The model under review builds one solid part; all positions refer to its coordinate system, in mm. Face numbers are marked on the shaded views. A direction names the side the tool comes from. Round coordinates to 2 decimals unless told otherwise and drop trailing zeros. Write each loop counter-clockwise with the first axis right and the second up, starting at its lowest first coordinate (ties: lowest second). Pieces come first, ordered by that corner, then holes. Notation, with made-up numbers: (-18.5, 52) -> (9.5, 52) arc R20 ccw to (9.5, 89) -> close; hole circle Ø6 at (-40, 57.25). An arc over 180 degrees is marked (long way). Answer as a JSON object with one key per item and string values. Group by question number.
1) To check wall thickness, follow probe 1 along X at (y, z) = (-14.5, 26); probe 2 along X at (y, z) = (-7, 34); probe 3 along X at (y, z) = (-9.5, 32). State the ranges of each line that lie inside material, in increasing order. Write a range as [from, to].
2) We need section B-B, the plane x = -68. Write out the cut boundary in (y, z), then the cut area to 3 significant figures.
3) Mouldability with a two-part tool opening along X and no side actions: class the marked faces 1, 2 and 3 as pulls with the +X half, pulls with the -X half, needs draft (parallel to the pull), parting line crosses it, or undercut.
4) We need section A-A, the plane z = -8. Write out the cut boundary in (x, y).
5) Machinability: for the marked faces 4 and 5, which of the approach directions +Z, -Z, +X, -X, +Y, -Y give a long, thin tool a straight path to every point of the face, cutting with its end or side? Answer none if there is none.
6) Insertion check: pin 1 Ø12 at (y, z) = (2.5, 37) entering from -X; pin 2 Ø6 at (y, z) = (-2.5, 6) entering from +X; pin 3 Ø8 at (x, z) = (-57.5, -28) entering from +Y. Each pin has a flat end and moves straight along its axis. Give the tip position at first contact, or say it passes through.
7) We need section C-C, the plane x = 32.5. Write out the cut boundary in (y, z).
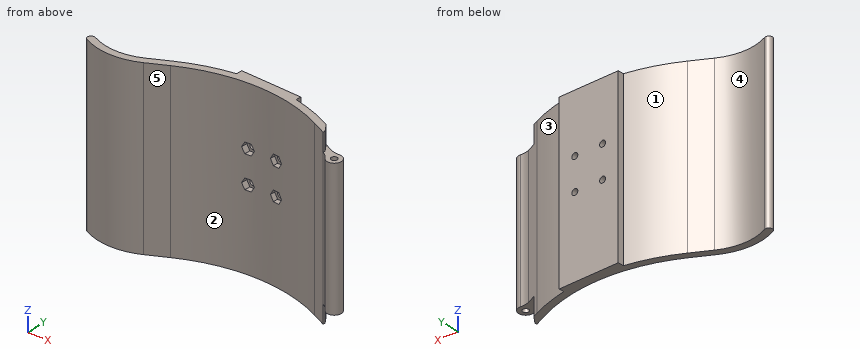
from build123d import *

# Parameters (mm, degrees)
CROQUIS1_R                   = 1.7
SALIENTE_EXTRUIR1_DEPTH      = 48
REDONDEO1_R                  = 10
CORTAR_EXTRUIR1_DEPTH        = 10
CHAFL_N1_SIZE                = 3
CHAFL_N1_SIZE2               = 5.196152423
CHAFL_N1_PART_2_SIZE         = 3
CHAFL_N1_PART_2_SIZE2        = 5.196152423
SALIENTE_EXTRUIR2_DEPTH      = 48
SALIENTE_EXTRUIR2_DEPTH_BACK = 48
CORTAR_EXTRUIR3_REACH        = 30.364
CROQUIS6_R                   = 1.7
CORTAR_EXTRUIR4_REACH        = 27.364


with BuildPart() as part:
    # Croquis1 → Saliente-Extruir1 (new body, symmetric)
    with BuildSketch(Plane.XY):
        with BuildLine():
            Line((-39.737417582, -9.247677161), (-50.50439396, -14.545999505))
            ThreePointArc((-50.50439396, -14.545999505), (-66.386844231, -18.110333527), (-82.148948738, -14.04674335))
            ThreePointArc((-82.148948738, -14.04674335), (-82.975471065, -11.341773693), (-80.270501408, -10.515251366))
            ThreePointArc((-80.270501408, -10.515251366), (-66.323744082, -14.110831262), (-52.270501408, -10.957007379))
            Line((-52.270501408, -10.957007379), (-41.50352503, -5.658685035))
            ThreePointArc((-41.50352503, -5.658685035), (0, 4), (41.50352503, -5.658685035))
            Line((41.50352503, -5.658685035), (52.270501408, -10.957007379))
            ThreePointArc((52.270501408, -10.957007379), (58.084598166, -16.047104806), (50.50439396, -14.545999505))
            Line((50.50439396, -14.545999505), (39.737417582, -9.247677161))
            ThreePointArc((39.737417582, -9.247677161), (0, 0), (-39.737417582, -9.247677161))
        make_face()
        with Locations((54.49560604, -14.280997358)):
            Circle(CROQUIS1_R, mode=Mode.SUBTRACT)
    extrude(amount=SALIENTE_EXTRUIR1_DEPTH, both=True)

    # Redondeo1
    redondeo1_edges = [part.edges().sort_by_distance(p)[0] for p in [
        (52.270501408, -10.957007379, 0),
        (50.50439396, -14.545999505, 0),
    ]]
    fillet(redondeo1_edges, radius=REDONDEO1_R)

    # Croquis3 → Cortar-Extruir1 (cut)
    with BuildSketch(Plane.XY.offset(48)):
        with BuildLine():
            Line((48.908512195, -9.302605814), (47.142404747, -12.89159794))
            ThreePointArc((47.142404747, -12.89159794), (49.37979166, -14.398010057), (51.133186064, -16.4475919))
            ThreePointArc((51.133186064, -16.4475919), (58.084598166, -16.047104806), (54.160798833, -10.295033969))
            ThreePointArc((54.160798833, -10.295033969), (51.467117745, -10.156254046), (48.908512195, -9.302605814))
        make_face()
    cortar_extruir1 = extrude(amount=-CORTAR_EXTRUIR1_DEPTH, mode=Mode.SUBTRACT)

    # Simetría1: Cortar-Extruir1 across plane
    add(cortar_extruir1.mirror(Plane.XY), mode=Mode.SUBTRACT)

    # Chaflán1
    chafl_n1_edges = [part.edges().sort_by_distance(p)[0] for p in [
        (48.908512195, -9.302605814, 43),
    ]]
    chafl_n1_side = [part.faces().sort_by_distance(p)[0] for p in [
        (48.025458471, -11.097101877, 43),
    ]]
    chamfer(chafl_n1_edges, length=CHAFL_N1_SIZE, length2=CHAFL_N1_SIZE2, reference=chafl_n1_side[0])

    # Chaflán1 part 2
    chafl_n1_part_2_edges = [part.edges().sort_by_distance(p)[0] for p in [
        (48.908512195, -9.302605814, -43),
    ]]
    chafl_n1_part_2_side = [part.faces().sort_by_distance(p)[0] for p in [
        (48.025458471, -11.097101877, -43),
    ]]
    chamfer(chafl_n1_part_2_edges, length=CHAFL_N1_PART_2_SIZE, length2=CHAFL_N1_PART_2_SIZE2, reference=chafl_n1_part_2_side[0])

    # Croquis5 → Saliente-Extruir2 (add, two sides)
    with BuildSketch(Plane.XY) as saliente_extruir2_sk:
        with BuildLine():
            Line((-12.976702091, 6.440682618), (20.976702091, 4.661260106))
            Line((20.976702091, 4.661260106), (20.819694222, 1.665371501))
            ThreePointArc((20.819694222, 1.665371501), (3.897584771, 3.91916116), (-13.153078528, 3.075219716))
            Line((-13.153078528, 3.075219716), (-12.976702091, 6.440682618))
        make_face()
    extrude(amount=SALIENTE_EXTRUIR2_DEPTH)
    extrude(saliente_extruir2_sk.sketch, amount=-SALIENTE_EXTRUIR2_DEPTH_BACK)

    # Croquis6 → Cortar-Extruir3 (cut, up to next)
    with BuildSketch(Plane(origin=(0.301073462, 5.744823887, 0), x_dir=(0.998629535, -0.052335956, 0), z_dir=(0.052335956, 0.998629535, 0)), mode=Mode.PRIVATE) as cortar_extruir3_sk1:
        with Locations((-4.295997255, 3)):
            Circle(CROQUIS6_R)
    cortar_extruir3_tool1 = extrude(cortar_extruir3_sk1.sketch, amount=-CORTAR_EXTRUIR3_REACH, mode=Mode.PRIVATE) & part.part
    add(cortar_extruir3_tool1.solids().sort_by_distance((-3.989036, 5.969659, -3))[0], mode=Mode.SUBTRACT)
    # Croquis6 → Cortar-Extruir3 (cut, up to next)
    with BuildSketch(Plane(origin=(0.301073462, 5.744823887, 0), x_dir=(0.998629535, -0.052335956, 0), z_dir=(0.052335956, 0.998629535, 0)), mode=Mode.PRIVATE) as cortar_extruir3_sk2:
        with Locations((11.704002745, 3)):
            Circle(CROQUIS6_R)
    cortar_extruir3_tool2 = extrude(cortar_extruir3_sk2.sketch, amount=-CORTAR_EXTRUIR3_REACH, mode=Mode.PRIVATE) & part.part
    add(cortar_extruir3_tool2.solids().sort_by_distance((11.989036, 5.132284, -3))[0], mode=Mode.SUBTRACT)
    # Croquis6 → Cortar-Extruir3 (cut, up to next)
    with BuildSketch(Plane(origin=(0.301073462, 5.744823887, 0), x_dir=(0.998629535, -0.052335956, 0), z_dir=(0.052335956, 0.998629535, 0)), mode=Mode.PRIVATE) as cortar_extruir3_sk3:
        with Locations((11.704002745, -15)):
            Circle(CROQUIS6_R)
    cortar_extruir3_tool3 = extrude(cortar_extruir3_sk3.sketch, amount=-CORTAR_EXTRUIR3_REACH, mode=Mode.PRIVATE) & part.part
    add(cortar_extruir3_tool3.solids().sort_by_distance((11.989036, 5.132284, 15))[0], mode=Mode.SUBTRACT)
    # Croquis6 → Cortar-Extruir3 (cut, up to next)
    with BuildSketch(Plane(origin=(0.301073462, 5.744823887, 0), x_dir=(0.998629535, -0.052335956, 0), z_dir=(0.052335956, 0.998629535, 0)), mode=Mode.PRIVATE) as cortar_extruir3_sk4:
        with Locations((-4.295997255, -15)):
            Circle(CROQUIS6_R)
    cortar_extruir3_tool4 = extrude(cortar_extruir3_sk4.sketch, amount=-CORTAR_EXTRUIR3_REACH, mode=Mode.PRIVATE) & part.part
    add(cortar_extruir3_tool4.solids().sort_by_distance((-3.989036, 5.969659, 15))[0], mode=Mode.SUBTRACT)

    # Croquis7 → Cortar-Extruir4 (cut, up to next)
    with BuildSketch(Plane(origin=(0.144065594, 2.748935283, 0), x_dir=(0.998629535, -0.052335956, 0), z_dir=(0.052335956, 0.998629535, 0)), mode=Mode.PRIVATE) as cortar_extruir4_sk1:
        Polygon((-0.889630667, 3), (-2.592813961, 5.95), (-5.999180549, 5.95), (-7.702363843, 3), (-5.999180549, 0.05), (-2.592813961, 0.05), align=None)
    cortar_extruir4_tool1 = extrude(cortar_extruir4_sk1.sketch, amount=-CORTAR_EXTRUIR4_REACH, mode=Mode.PRIVATE) & part.part
    add(cortar_extruir4_tool1.solids().sort_by_distance((-4.146044, 2.97377, -3))[0], mode=Mode.SUBTRACT)
    # Croquis7 → Cortar-Extruir4 (cut, up to next)
    with BuildSketch(Plane(origin=(0.144065594, 2.748935283, 0), x_dir=(0.998629535, -0.052335956, 0), z_dir=(0.052335956, 0.998629535, 0)), mode=Mode.PRIVATE) as cortar_extruir4_sk2:
        Polygon((15.110369333, 3), (13.407186039, 5.95), (10.000819451, 5.95), (8.297636157, 3), (10.000819451, 0.05), (13.407186039, 0.05), align=None)
    cortar_extruir4_tool2 = extrude(cortar_extruir4_sk2.sketch, amount=-CORTAR_EXTRUIR4_REACH, mode=Mode.PRIVATE) & part.part
    add(cortar_extruir4_tool2.solids().sort_by_distance((11.832028, 2.136395, -3))[0], mode=Mode.SUBTRACT)
    # Croquis7 → Cortar-Extruir4 (cut, up to next)
    with BuildSketch(Plane(origin=(0.144065594, 2.748935283, 0), x_dir=(0.998629535, -0.052335956, 0), z_dir=(0.052335956, 0.998629535, 0)), mode=Mode.PRIVATE) as cortar_extruir4_sk3:
        Polygon((-0.889630667, -15), (-2.592813961, -12.05), (-5.999180549, -12.05), (-7.702363843, -15), (-5.999180549, -17.95), (-2.592813961, -17.95), align=None)
    cortar_extruir4_tool3 = extrude(cortar_extruir4_sk3.sketch, amount=-CORTAR_EXTRUIR4_REACH, mode=Mode.PRIVATE) & part.part
    add(cortar_extruir4_tool3.solids().sort_by_distance((-4.146044, 2.97377, 15))[0], mode=Mode.SUBTRACT)
    # Croquis7 → Cortar-Extruir4 (cut, up to next)
    with BuildSketch(Plane(origin=(0.144065594, 2.748935283, 0), x_dir=(0.998629535, -0.052335956, 0), z_dir=(0.052335956, 0.998629535, 0)), mode=Mode.PRIVATE) as cortar_extruir4_sk4:
        Polygon((15.110369333, -15), (13.407186039, -12.05), (10.000819451, -12.05), (8.297636157, -15), (10.000819451, -17.95), (13.407186039, -17.95), align=None)
    cortar_extruir4_tool4 = extrude(cortar_extruir4_sk4.sketch, amount=-CORTAR_EXTRUIR4_REACH, mode=Mode.PRIVATE) & part.part
    add(cortar_extruir4_tool4.solids().sort_by_distance((11.832028, 2.136395, 15))[0], mode=Mode.SUBTRACT)


solid = part.part
Here are the results:
{
 "1": {"probe 1": "x = [-81.27, -50.41], [49.49, 52.81], [56.18, 58.49]", "probe 2": "x = [-44.23, -34.8], [34.8, 44.23]", "probe 3": "x = [-49.31, -40.25], [40.25, 49.33]"},
 "2": {"outline": "(-18.05, -48) -> (-14.04, -48) -> (-14.04, 48) -> (-18.05, 48) -> close", "area": "385 mm^2"},
 "3": {"face 1": "pulls with the -X half", "face 2": "undercut", "face 3": "pulls with the +X half"},
 "4": {"outline": "(-82.15, -14.05) arc R34.73 ccw to (-50.5, -14.55) -> (-39.74, -9.25) arc R90 cw to (39.74, -9.25) -> (47.14, -12.89) arc R10 cw to (51.13, -16.45) arc R4 ccw (long way) to (54.16, -10.3) arc R10 cw to (48.91, -9.3) -> (41.5, -5.66) arc R94 ccw to (20.82, 1.67) -> (20.98, 4.66) -> (-12.98, 6.44) -> (-13.15, 3.08) arc R94 ccw to (-41.5, -5.66) -> (-52.27, -10.96) arc R30.73 cw to (-80.27, -10.52) arc R2 ccw to start; hole circle Ø3.4 at (54.5, -14.28)"},
 "5": {"face 4": "+Z, -Z, +Y", "face 5": "+Z, -Z, -Y"},
 "6": {"pin 1": "stops at x = -36.79", "pin 2": "stops at x = 41.18", "pin 3": "stops at y = -11.53"},
 "7": {"outline": "(-6.07, -48) -> (-1.8, -48) -> (-1.8, 48) -> (-6.07, 48) -> close"}
}
